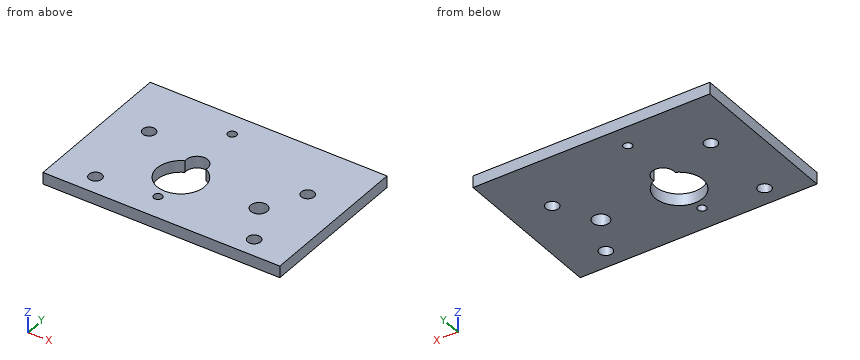
```python
from build123d import *

# Parameters (mm, degrees)
SKETCH_1_W          = 60.6
SKETCH_1_H          = 40
EXTRUDE_1_DEPTH     = 3
SKETCH_2_R          = 2.75
SKETCH_2_R_2        = 6.1
SKETCH_2_R_3        = 1.1
SKETCH_2_R_4        = 2.1
CUT_EXTRUDE_1_DEPTH = 73.672966088
SKETCH_3_R          = 1.65
CUT_EXTRUDE_2_DEPTH = 13


with BuildPart() as part:
    # 草图1 → 凸台-拉伸1 (new body)
    with BuildSketch(Plane.XY):
        with Locations((30.3, 20)):
            Rectangle(SKETCH_1_W, SKETCH_1_H)
    extrude(amount=EXTRUDE_1_DEPTH)

    # 草图2 → 切除-拉伸1 (cut, through all)
    with BuildSketch(Plane(origin=(0, 0, 0), x_dir=(-1, 0, 0), z_dir=(0, 0, -1))):
        with Locations((-25, 21)):
            Circle(SKETCH_2_R)
        with Locations((-25, 15)):
            Circle(SKETCH_2_R_2)
        with Locations((-25, 6.46)):
            Circle(SKETCH_2_R_3)
        with Locations((-25, 34.14)):
            Circle(SKETCH_2_R_3)
        with Locations((-45, 15)):
            Circle(SKETCH_2_R_4)
    extrude(amount=-CUT_EXTRUDE_1_DEPTH, mode=Mode.SUBTRACT)

    # 草图3 → 切除-拉伸2 (cut)
    with BuildSketch(Plane.XY.offset(3)):
        with Locations((50.6, 5)):
            Circle(SKETCH_3_R)
        with Locations((50.6, 25)):
            Circle(SKETCH_3_R)
        with Locations((10, 25)):
            Circle(SKETCH_3_R)
        with Locations((10, 5)):
            Circle(SKETCH_3_R)
    extrude(amount=-CUT_EXTRUDE_2_DEPTH, mode=Mode.SUBTRACT)


solid = part.part
```
Geometry check sheet. Reference: the model listing, model coordinates, mm. Give positions to 0.01 mm unless a question says otherwise; leave off trailing zeros. Write each loop counter-clockwise with the first axis right and the second up, starting at its lowest first coordinate (ties: lowest second). Pieces come first, ordered by that corner, then holes.
1) Section check B-B, the plane x = 50.6. Record the boundary of the cut face in (y, z).
2) Section check C-C, the plane x = 25. Record the boundary of the cut face in (y, z), and give its area (4 significant figures).
3) Section check D-D, the plane y = 34.14. Record the boundary of the cut face in (x, z), and give its area (3 significant figures).
4) Gauge pin test, flat end, axial feed: pin 1 (11 mm diameter, centred on x = 25, y = 15, fed in from +Z). Record the tip position at first contact, or that the pin passes through.
5) Section check A-A, the plane y = 25. Record the boundary of the cut face in (x, z).
6) Material ranges on L1, parallel to Y at x = 10, z = 1.2; L2, parallel to Y at x = 45, z = 2.45; L3, parallel to X at y = 21, z = 0.7, recorded low to high.
Computed:
1. outline: (0, 0) - (3.35, 0) - (3.35, 3) - (0, 3) - close; (6.65, 0) - (23.35, 0) - (23.35, 3) - (6.65, 3) - close; (26.65, 0) - (40, 0) - (40, 3) - (26.65, 3) - close
2. outline: (0, 0) - (5.36, 0) - (5.36, 3) - (0, 3) - close; (7.56, 0) - (8.9, 0) - (8.9, 3) - (7.56, 3) - close; (23.75, 0) - (33.04, 0) - (33.04, 3) - (23.75, 3) - close; (35.24, 0) - (40, 0) - (40, 3) - (35.24, 3) - close
2. area: 62.25 mm2
3. outline: (0, 0) - (23.9, 0) - (23.9, 3) - (0, 3) - close; (26.1, 0) - (60.6, 0) - (60.6, 3) - (26.1, 3) - close
3. area: 175 mm2
4. pin 1: passes through
5. outline: (0, 0) - (8.35, 0) - (8.35, 3) - (0, 3) - close; (11.65, 0) - (48.95, 0) - (48.95, 3) - (11.65, 3) - close; (52.25, 0) - (60.6, 0) - (60.6, 3) - (52.25, 3) - close
6. L1: y = 0 to 3.35, 6.65 to 23.35, 26.65 to 40
6. L2: y = 0 to 12.9, 17.1 to 40
6. L3: x = 0 to 22.25, 27.75 to 60.6
